from build123d import *

# Parameters (mm, degrees)
F0_R      = 114
F0_R_2    = 9.5
F1_DEPTH  = 25
F2_R      = 50
F3_DEPTH  = 60
F4_R      = 22.5
F5_DEPTH  = 450
F6_W      = 100
F6_H      = 100
F7_DEPTH  = 100
F8_R      = 15
F9_DEPTH  = 50
F10_R     = 44.188125
F11_DEPTH = 300
F12_W     = 74.58368
F12_H     = 105.065704
F13_DEPTH = 10


with BuildPart() as f1:
    # F0 (on Front) → F1 (new body)
    with BuildSketch(Plane.XZ):
        Circle(F0_R)
        with Locations((-67.175144, -67.175144)):
            Circle(F0_R_2, mode=Mode.SUBTRACT)
        with Locations((0, -95)):
            Circle(F0_R_2, mode=Mode.SUBTRACT)
        with Locations((67.175144, -67.175144)):
            Circle(F0_R_2, mode=Mode.SUBTRACT)
        with Locations((-95, 0)):
            Circle(F0_R_2, mode=Mode.SUBTRACT)
        with Locations((-67.175144, 67.175144)):
            Circle(F0_R_2, mode=Mode.SUBTRACT)
        with Locations((95, 0)):
            Circle(F0_R_2, mode=Mode.SUBTRACT)
        with Locations((0, 95)):
            Circle(F0_R_2, mode=Mode.SUBTRACT)
        with Locations((67.175144, 67.175144)):
            Circle(F0_R_2, mode=Mode.SUBTRACT)
    extrude(amount=F1_DEPTH)

    # F2 (on face) → F3 (join)
    with BuildSketch(Plane.XZ.offset(25)):
        Circle(F2_R)
    extrude(amount=F3_DEPTH)

    # F4 (on face) → F5 (join)
    with BuildSketch(Plane.XZ.offset(85)):
        Circle(F4_R)
    extrude(amount=F5_DEPTH)

    # F6 (on face) → F7 (join)
    with BuildSketch(Plane.XZ.offset(535)):
        Rectangle(F6_W, F6_H)
    extrude(amount=F7_DEPTH)

    # F8 (on face) → F9 (join)
    with BuildSketch(Plane(origin=(0, 0, -50), x_dir=(1, 0, 0), z_dir=(0, 0, -1))):
        with Locations((0, 585)):
            Circle(F8_R)
    extrude(amount=F9_DEPTH)

    # F10 (on face) → F11 (join)
    with BuildSketch(Plane(origin=(0, 0, -100), x_dir=(1, 0, 0), z_dir=(0, 0, -1))):
        with Locations((0, 585)):
            Circle(F10_R)
    extrude(amount=F11_DEPTH)

    # F12 (on Right) → F13 (join, symmetric)
    with BuildSketch(Plane.YZ):
        with Locations((-512.605652, -333.903551)):
            Rectangle(F12_W, F12_H)
    extrude(amount=F13_DEPTH, both=True)


solid = f1.part
Could you check a few things on this model? Use its own coordinates, in mm. A direction names the side the tool comes from. Coordinates: 2 decimals unless noted, no trailing zeros. Order: outer loops, then holes, each group sorted by start corner. A loop starts at its lowest first (then second) coordinate and runs counter-clockwise, first axis right, second up.
Q1. Suppose I cut it at B-B on x = 95. Please give me the cut outline in (y, z), and give its area (3 significant figures).
Q2. Suppose I cut it at C-C on y = -511.5. Please give me the cut outline in (x, z).
Q3. Suppose I cut it at D-D on z = 95. Please give me the cut outline in (x, y).
Q4. Suppose I cut it at A-A on z = 0. Please give me the cut outline in (x, y), and give its area (3 significant figures).
Q5. Will these pins go through, and if not, where does the flat tip stop? pin 1 (10 mm diameter, centred on x = -4.5, y = -515, fed in from -Z); pin 2 (22 mm diameter, centred on x = 0, z = -95, fed in from -Y); pin 3 (22 mm diameter, centred on x = 2, z = -318, fed in from +Y).
Q6. Please list where these lines run through material, in increasing order: L1, parallel to Y at x = -46, z = -47.5; L2, parallel to Z at x = -35.5, y = -572.5; L3, parallel to Y at x = 46, z = 8.5.
Q7. Which directions (+Z, -Z, +X, -X, +Y, -Y) give clear straight access to the entire face, cutting with the end or side of a thin tool? Please do faces 1 (the flat face through (-10, -509, -333)), 2 (the cylindrical face through (-1.24, -12.32, -85.58)), 3 (the flat face through (10, -85, -22)).
Q8. Thinking about a two-plate mould opening in Y: for faces 4 (the cylindrical face through (60.173, -12.325, 73.596)), 5 (the cylindrical face through (10.382, -306.85, -19.961)), 6 (the flat face through (-1, -635, 1)), which applies, released by +Y, released by -Y, zero draft, split by the parting line, or undercut?
Answer:
1. outline: (-25, -63.02) - (0, -63.02) - (0, -9.5) - (-25, -9.5) - close; (-25, 9.5) - (0, 9.5) - (0, 63.02) - (-25, 63.02) - close
1. area: 2,680 mm2
2. outline: circle Ø45 at (0, 0); (-10, -386.44) - (10, -386.44) - (10, -281.37) - (-10, -281.37) - close
3. outline: (-63.02, -25) - (-9.5, -25) - (-9.5, 0) - (-63.02, 0) - close; (9.5, -25) - (63.02, -25) - (63.02, 0) - (9.5, 0) - close
4. outline: (-114, -25) - (-104.5, -25) - (-104.5, 0) - (-114, 0) - close; (-85.5, -25) - (-50, -25) - (-50, -85) - (-22.5, -85) - (-22.5, -535) - (-50, -535) - (-50, -635) - (50, -635) - (50, -535) - (22.5, -535) - (22.5, -85) - (50, -85) - (50, -25) - (85.5, -25) - (85.5, 0) - (-85.5, 0) - close; (104.5, -25) - (114, -25) - (114, 0) - (104.5, 0) - close
4. area: 41,000 mm2
5. pin 1: stops at z = -386.44
5. pin 2: stops at y = -629.19
5. pin 3: stops at y = -475.31
6. L1: y = -635 to -535, -25 to 0
6. L2: z = -400 to -100, -50 to 50
6. L3: y = -635 to -535, -85 to 0
7. face 1: -Z, -X, +Y
7. face 2: +Y
7. face 3: none
8. face 4: zero draft
8. face 5: undercut
8. face 6: released by -Y
